```python
from build123d import *

# Parameters (mm, degrees)
SKETCH_1_W                   = 153
SKETCH_1_H                   = 45
SKETCH_1_R                   = 10
SKETCH_1_R_2                 = 4.25
EXTRUDE_1_DEPTH              = 5
SKETCH_6_R                   = 12
CUT_EXTRUDE_1028_DEPTH       = 8
CHAMFER_1_SIZE               = 5
FILLET_1_R                   = 5
CHAMFER_2_SIZE               = 0.2
HOLE_WIZARD_M4_1_D           = 3.3
HOLE_WIZARD_M4_1_DEPTH       = 15.5
HOLE_WIZARD_M4_1_CSINK_D     = 4.05
HOLE_WIZARD_M4_1_CSINK_ANGLE = 120


with BuildPart() as part:
    # 草图1 → 凸台-拉伸1 (new body, symmetric)
    with BuildSketch(Plane(origin=(0, 0, 0), x_dir=(0, 0, -1), z_dir=(1, 0, 0))):
        with Locations((76.5, -22.5)):
            Rectangle(SKETCH_1_W, SKETCH_1_H)
        with Locations((28.5, -22.5)):
            Circle(SKETCH_1_R, mode=Mode.SUBTRACT)
        with Locations((85.5, -22.5)):
            Circle(SKETCH_1_R_2, mode=Mode.SUBTRACT)
        with Locations((130.5, -22.5)):
            Circle(SKETCH_1_R_2, mode=Mode.SUBTRACT)
    extrude(amount=EXTRUDE_1_DEPTH, both=True)

    # 草图6 → Cut-Extrude 1028 (cut)
    with BuildSketch(Plane.ZY.offset(-5)):
        with Locations((-28.5, -22.5)):
            Circle(SKETCH_6_R)
    extrude(amount=CUT_EXTRUDE_1028_DEPTH, mode=Mode.SUBTRACT)

    # 倒角1
    chamfer_1_edges = [part.edges().sort_by_distance(p)[0] for p in [
        (0, 0, -153),
        (0, -45, -153),
    ]]
    chamfer(chamfer_1_edges, length=CHAMFER_1_SIZE)

    # 圆角1
    fillet_1_edges = [part.edges().sort_by_distance(p)[0] for p in [
        (0, 0, 0),
        (0, -45, 0),
    ]]
    fillet(fillet_1_edges, radius=FILLET_1_R)

    # 倒角2
    chamfer_2_edges = [part.edges().sort_by_distance(p)[0] for p in [
        (5, -22.5, -40.5),
    ]]
    chamfer(chamfer_2_edges, length=CHAMFER_2_SIZE)

    # M4 螺纹孔1
    with Locations(Plane.XY):
        with Locations((0, -10), (0, -35)):
            CounterSinkHole(HOLE_WIZARD_M4_1_D / 2, HOLE_WIZARD_M4_1_CSINK_D / 2, depth=HOLE_WIZARD_M4_1_DEPTH, counter_sink_angle=HOLE_WIZARD_M4_1_CSINK_ANGLE)


solid = part.part
```
The listing builds one solid part. Answer for the finished solid, in the listing's coordinates (mm). A direction names the side the tool comes from. Round coordinates to 2 decimals unless told otherwise and drop trailing zeros. Write each loop counter-clockwise with the first axis right and the second up, starting at its lowest first coordinate (ties: lowest second). Pieces come first, ordered by that corner, then holes. Notation, with made-up numbers: (37.25, 23.5) -> (50.25, 23.5) arc R7 cw to (50.25, 36.5) -> close; hole circle Ø2 at (-28.5, -17.75). An arc over 180 degrees is marked (long way). Answer as a JSON object with one key per item and string values. Group by question number.
Q1. Section A-A (y = -22.5) is taken. Write down the section's boundary in (x, z), plus the area to 3 significant figures.
Q2. Section B-B (z = -85.5) is taken. Write down the section's boundary in (x, y).
Q3. Determine the mould class of faces 1 (the face through (0, -42, -151)), 2 (the face through (-5, -22, -75)), 3 (the face through (0.955, -18.896, -17.054)), 4 (the face through (-0.89, -33.61, -7.97)) for opening direction Y: pulls with the +Y half, pulls with the -Y half, needs draft (parallel to the pull), parting line crosses it, or undercut.
Q4. Each of these flat-tipped pins is pushed along its axis until it touches: pin 1 Ø11 at (y, z) = (-22.5, -130.5) entering from +X; pin 2 Ø3 at (x, y) = (0, -35) entering from +Z; pin 3 Ø7 at (y, z) = (-17.5, -33) entering from +X; pin 4 Ø19 at (y, z) = (-22.5, -28.5) entering from -X. Where does it stop, or does it pass through?
Q5. Section D-D (z = -28.5) is taken. Write down the section's boundary in (x, y), plus the area to 3 significant figures.
Q6. Which of the six approach directions +Z, -Z, +X, -X, +Y, -Y give full straight-line access (tool end or side, diameter ignored) to faces 5 (the face through (0, -45, -75)), 6 (the face through (-3, -12.7, -31.2)), 7 (the face through (0, -10, -15.5))?
Q7. Straight lines are drawn through the part: line 1 along Z through (x, y) = (2, -23); line 2 along Y through (x, z) = (-4, -28.5); line 3 along Y through (x, z) = (1.5, -85.5). For each, find the intervals that lie inside material, in ascending order.
Q8. Section C-C (x = 0) is taken. Count the separate pieces of the cut face and the enclosed holes in it, plus the area to 3 significant figures.
Check values:
{
 "1": {"outline": "(-5, -153) -> (5, -153) -> (5, -134.75) -> (-5, -134.75) -> close; (-5, -126.25) -> (5, -126.25) -> (5, -89.75) -> (-5, -89.75) -> close; (-5, -81.25) -> (5, -81.25) -> (5, -40.7) -> (4.8, -40.5) -> (-3, -40.5) -> (-3, -38.5) -> (-5, -38.5) -> close; (-5, -18.5) -> (-3, -18.5) -> (-3, -16.5) -> (4.8, -16.5) -> (5, -16.3) -> (5, 0) -> (-5, 0) -> close", "area": "1,130 mm^2"},
 "2": {"outline": "(-5, -45) -> (5, -45) -> (5, -26.75) -> (-5, -26.75) -> close; (-5, -18.25) -> (5, -18.25) -> (5, 0) -> (-5, 0) -> close"},
 "3": {"face 1": "pulls with the -Y half", "face 2": "needs draft", "face 3": "undercut", "face 4": "undercut"},
 "4": {"pin 1": "x = 5", "pin 2": "z = -15.5", "pin 3": "x = -3", "pin 4": "through"},
 "5": {"outline": "(-5, -45) -> (5, -45) -> (5, -34.7) -> (4.8, -34.5) -> (-3, -34.5) -> (-3, -32.5) -> (-5, -32.5) -> close; (-5, -12.5) -> (-3, -12.5) -> (-3, -10.5) -> (4.8, -10.5) -> (5, -10.3) -> (5, 0) -> (-5, 0) -> close", "area": "218 mm^2"},
 "6": {"face 5": "+Z, -Z, +X, -X, -Y", "face 6": "+X", "face 7": "+Z"},
 "7": {"line 1": "-153 to -134.72, -126.28 to -89.72, -81.28 to -40.49, -16.51 to 0", "line 2": "-45 to -32.5, -12.5 to 0", "line 3": "-45 to -26.75, -18.25 to 0"},
 "8": {"separate pieces": "1", "enclosed holes": "3", "area": "6,180 mm^2"}
}
